Source: CAD feature listing. Evaluate the final solid. Frame: model axes, mm. Coordinates: 2 decimals unless noted, no trailing zeros. Order: outer loops, then holes, each group sorted by start corner. A loop starts at its lowest first (then second) coordinate and runs counter-clockwise, first axis right, second up. Notation, with made-up numbers: (70.5, 33.5) - (115.5, 33.5) arc R24 ccw to (115.5, 50.5) - close; hole circle Ø5 at (-1.75, 13). An arc over 180 degrees is marked (long way). One line per question, with ' | ' between items. Start each with the question number.
(1) Section A-A (x = 5). Return the cut outline in (y, z).
(2) Section D-D (x = -12). Return the cut outline in (y, z).
(3) Contact query for a flat-ended pin moving along its axis: P1, Ø8, axis at x = -9, z = 28.5, coming from the +Y side. Output: stop coordinate, or through.
(4) Section C-C (y = -1.6). Return the cut outline in (x, z), then the cut area to 3 significant figures.
(5) Line query: line 1 along X through (y, z) = (-0.55, 38.5); line 2 along X through (y, z) = (-1.5, 45); line 3 along Z through (x, y) = (-4, -0.05). Output: solid intervals per line, ascending.
(6) Section B-B (z = 51.5). Return the cut outline in (x, y), then the cut area to 3 significant figures.
from build123d import *

# Parameters (mm, degrees)
F1_DEPTH = 2.5


with BuildPart() as f1:
    # F0 (on Front) → F1 (new body)
    with BuildSketch(Plane.XZ):
        with BuildLine():
            ThreePointArc((10, 46.943923), (-7.071068, 54.01499), (0, 36.943923))
            ThreePointArc((0, 36.943923), (7.071068, 39.872855), (10, 46.943923))
        make_face()
        with BuildLine():
            Line((-16.124446, 0), (0, 0))
            Line((0, 0), (16.124446, 0))
            Line((16.124446, 0), (16.124446, 46.943923))
            ThreePointArc((16.124446, 46.943923), (0, 63.068368), (-16.124446, 46.943923))
            Line((-16.124446, 46.943923), (-16.124446, 0))
        make_face()
        with BuildLine():
            ThreePointArc((10, 46.943923), (7.071068, 39.872855), (0, 36.943923))
            ThreePointArc((0, 36.943923), (-7.071068, 54.01499), (10, 46.943923))
        make_face(mode=Mode.SUBTRACT)
    extrude(amount=F1_DEPTH)


solid = f1.part
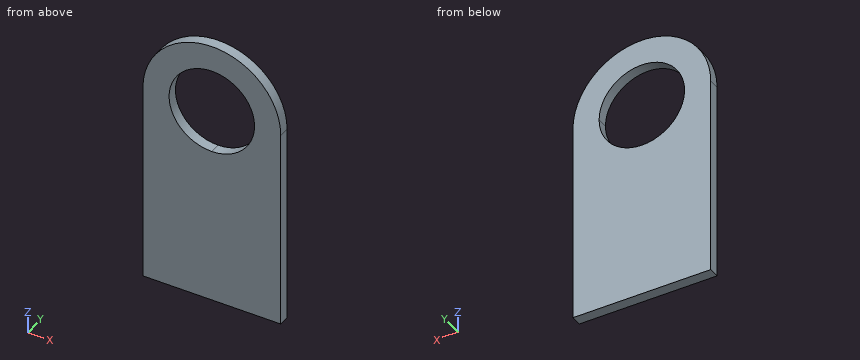
Response values:
1) outline: (-2.5, 0) - (0, 0) - (0, 38.28) - (-2.5, 38.28) - close; (-2.5, 55.6) - (0, 55.6) - (0, 62.27) - (-2.5, 62.27) - close
2) outline: (-2.5, 0) - (0, 0) - (0, 57.71) - (-2.5, 57.71) - close
3) P1: stops at y = 0
4) outline: (-16.12, 0) - (16.12, 0) - (16.12, 46.94) arc R16.12 ccw to (-16.12, 46.94) - close; hole circle Ø20 at (0, 46.94) | area: 1,610 mm²
5) line 1: x = -16.12 to -5.36, 5.36 to 16.12 | line 2: x = -16.12 to -9.81, 9.81 to 16.12 | line 3: z = 0 to 37.78, 56.11 to 62.56
6) outline: (-15.47, -2.5) - (-8.9, -2.5) - (-8.9, 0) - (-15.47, 0) - close; (8.9, -2.5) - (15.47, -2.5) - (15.47, 0) - (8.9, 0) - close | area: 32.8 mm²
